from build123d import *

# Parameters (mm, degrees)
SKETCH1_R               = 4
SKETCH1_R_2             = 2.5
BOSS_EXTRUDE1_DEPTH     = 1
BOSS_EXTRUDE1_2_DEPTH   = 1
BOSS_EXTRUDE2_START     = 1
BOSS_EXTRUDE2_DEPTH     = 0.5
CUT_EXTRUDE1_DEPTH      = 16.67695104
CUT_EXTRUDE1_DEPTH_BACK = 16.67695104
SKETCH4_R               = 1.5


with BuildPart() as part:
    # Sketch1 → Boss-Extrude1 (new, symmetric)
    with BuildSketch(Plane.XY):
        with Locations((-10.442114773, 0)):
            Circle(SKETCH1_R)
        with Locations((-10.442114773, 0)):
            Circle(SKETCH1_R_2, mode=Mode.SUBTRACT)
    extrude(amount=BOSS_EXTRUDE1_DEPTH, both=True)



with BuildPart() as body_2:
    # Sketch1 → Boss-Extrude1 2 (new, symmetric)
    with BuildSketch(Plane.XY):
        with Locations((3.557885227, 0)):
            Circle(SKETCH1_R)
        with Locations((3.557885227, 0)):
            Circle(SKETCH1_R_2, mode=Mode.SUBTRACT)
    extrude(amount=BOSS_EXTRUDE1_2_DEPTH, both=True)


with BuildPart() as part_1:
    add(part.part)

    add(body_2.part)  # Boss-Extrude2 merges body 2
    # Sketch2 → Boss-Extrude2 (add)
    with BuildSketch(Plane.XY.offset(BOSS_EXTRUDE2_START)):
        with BuildLine():
            ThreePointArc((-8.7771853, 4.180670981), (-14.942114773, 0), (-8.7771853, -4.180670981))
            ThreePointArc((-8.7771853, -4.180670981), (-3.442114773, -3.157418725), (1.892955754, -4.180670981))
            ThreePointArc((1.892955754, -4.180670981), (8.057885227, 0), (1.892955754, 4.180670981))
            ThreePointArc((1.892955754, 4.180670981), (-3.442114773, 3.157418725), (-8.7771853, 4.180670981))
        make_face()
    boss_extrude2 = extrude(amount=BOSS_EXTRUDE2_DEPTH)

    # Mirror1: Boss-Extrude2 across plane
    add(boss_extrude2.mirror(Plane.XY))

    # Sketch4 → Cut-Extrude1 (cut, two sides: drawn at the far end of the back side and taken through both)
    with BuildSketch(Plane.XY.offset(-CUT_EXTRUDE1_DEPTH_BACK)):
        with Locations((-10.442114773, 0)):
            Circle(SKETCH4_R)
        with Locations((3.557885227, 0)):
            Circle(SKETCH4_R)
    extrude(amount=CUT_EXTRUDE1_DEPTH + CUT_EXTRUDE1_DEPTH_BACK, mode=Mode.SUBTRACT)


solid = part_1.part
Geometry: final body of the model. Coordinates: model frame, mm. A direction names the side the tool comes from. Give positions to 0.01 mm unless a question says otherwise; leave off trailing zeros. Write each loop counter-clockwise with the first axis right and the second up, starting at its lowest first coordinate (ties: lowest second). Pieces come first, ordered by that corner, then holes.
(1) First-contact query: P1, Ø1.5, axis at y = -2.5, z = 1, coming from the +X side; P2, Ø1.5, axis at y = -2.5, z = 0, coming from the +X side. Flat tips, straight axial feed; report the tip coordinate or a pass-through.
(2) Cut plane D-D, the plane y = 3.5. Return loops of the section in (x, z), then the cut area to 3 significant figures.
(3) Mould query, pull axis Y, two halves, no side actions, for faces 1 (the cylindrical face through (2.06, 0.07, -1.25)), 2 (the cylindrical face through (-3.519, -3.158, 1.246)), 3 (the cylindrical face through (2.691, -3.905, 0.014)), 4 (the flat face through (-4, 0, 1.5)). Classes: released by +Y, released by -Y, zero draft, split by the parting line, or undercut.
(4) Cut plane C-C, the plane x = -2.25. Return loops of the section in (y, z).
(5) Ray query, line 1 (Z direction, x = -2, y = 3); line 2 (X direction, y = -1.25, z = -0.45); line 3 (X direction, y = -0.75, z = -1.3). Return the intervals inside material, ascending.
(6) Cut plane A-A, the plane y = 0. Give the number of separate pieces and of enclosed holes in the cut face, then the cut area to 3 significant figures.
(7) Access query for faces 5 (the flat face through (5, -1, 1)), 6 (the cylindrical face through (-3.366, 3.158, 1.246)). Directions: +Z, -Z, +X, -X, +Y, -Y. A direction counts if a zero-diameter tool reaches every point of the face in a straight line with its end or side. Return the directions, or none.
(8) Cut plane B-B, the plane z = -0.7. Return loops of the section in (x, y).
Values follow:
1. P1: stops at x = 7.7
1. P2: stops at x = 7.15
2. outline: (-13.27, -1.5) - (-6.57, -1.5) - (-6.57, -1) - (-8.51, -1) - (-8.51, 1) - (-6.57, 1) - (-6.57, 1.5) - (-13.27, 1.5) - (-13.27, 1) - (-12.38, 1) - (-12.38, -1) - (-13.27, -1) - close; (-0.32, -1.5) - (6.39, -1.5) - (6.39, -1) - (5.49, -1) - (5.49, 1) - (6.39, 1) - (6.39, 1.5) - (-0.32, 1.5) - (-0.32, 1) - (1.62, 1) - (1.62, -1) - (-0.32, -1) - close
2. area: 28.9 mm2
3. face 1: undercut
3. face 2: released by -Y
3. face 3: split by the parting line
3. face 4: zero draft
4. outline: (-3.21, -1.5) - (3.21, -1.5) - (3.21, -1) - (-3.21, -1) - close; (-3.21, 1) - (3.21, 1) - (3.21, 1.5) - (-3.21, 1.5) - close
5. line 1: z = -1.5 to -1, 1 to 1.5
5. line 2: x = -14.24 to -12.61, -8.28 to -6.64, -0.24 to 1.39, 5.72 to 7.36
5. line 3: x = -14.88 to -11.74, -9.14 to 2.26, 4.86 to 7.99
6. separate pieces: 3
6. enclosed holes: 1
6. area: 29.0 mm2
7. face 5: none
7. face 6: +Z, -Z, +Y
8. outline: circle Ø8 at (-10.44, 0); circle Ø8 at (3.56, 0); hole circle Ø5 at (-10.44, 0); hole circle Ø5 at (3.56, 0)
